Read the model definition and answer for the solid it produces. Units are mm, in the model's axes. Round coordinates to 2 decimals unless told otherwise and drop trailing zeros. Loops run counter-clockwise (first coordinate to the right, second up) from the corner with the lowest first, then second, coordinate; pieces in that order, holes last. Notation, with made-up numbers: M 9,-20.5 L 43,-20.5 A8 cw 43,-9.5 Z; hole C 24.25,-13.5 d1. An arc over 180 degrees is marked long. Write each question's results on one line, items separated by ' | '.
from build123d import *

# Parameters (mm, degrees)
SKETCH2_R           = 2.5
SKETCH2_R_2         = 250
BOSS_EXTRUDE1_DEPTH = 10
CUT_EXTRUDE1_DEPTH  = 11


with BuildPart() as part:
    # Sketch2 → Boss-Extrude1 (new body)
    with BuildSketch(Plane(origin=(0, 0, 0), x_dir=(1, 0, 0), z_dir=(0, 1, 0))):
        with BuildLine():
            Line((-34.517430478, 903.068960265), (-295.040344804, 95.1377682))
            ThreePointArc((-295.040344804, 95.1377682), (-310, 0), (-295.040344804, -95.1377682))
            Line((-295.040344804, -95.1377682), (-34.517430478, -903.068960265))
            ThreePointArc((-34.517430478, -903.068960265), (-30.886866626, -908.083613135), (-25, -910))
            Line((-25, -910), (25, -910))
            ThreePointArc((25, -910), (30.886866626, -908.083613135), (34.517430478, -903.068960265))
            Line((34.517430478, -903.068960265), (295.040344804, -95.1377682))
            ThreePointArc((295.040344804, -95.1377682), (310, 0), (295.040344804, 95.1377682))
            Line((295.040344804, 95.1377682), (34.517430478, 903.068960265))
            ThreePointArc((34.517430478, 903.068960265), (30.886866626, 908.083613135), (25, 910))
            Line((25, 910), (-25, 910))
            ThreePointArc((-25, 910), (-30.886866626, 908.083613135), (-34.517430478, 903.068960265))
        make_face()
        with Locations((-48.373467006, -762.345774842)):
            Circle(SKETCH2_R, mode=Mode.SUBTRACT)
        with Locations((-94.407870974, -619.584317679)):
            Circle(SKETCH2_R, mode=Mode.SUBTRACT)
        with Locations((-140.442274942, -476.822860516)):
            Circle(SKETCH2_R, mode=Mode.SUBTRACT)
        with BuildLine():
            ThreePointArc((-181.680791071, -251.181388952), (0, -310), (181.680791071, -251.181388952))
            Line((181.680791071, -251.181388952), (9.517430478, -785.092770658))
            ThreePointArc((9.517430478, -785.092770658), (0, -792.023810393), (-9.517430478, -785.092770658))
            Line((-9.517430478, -785.092770658), (-181.680791071, -251.181388952))
        make_face(mode=Mode.SUBTRACT)
        with Locations((-186.476678909, -334.061403353)):
            Circle(SKETCH2_R, mode=Mode.SUBTRACT)
        with Locations((48.373467006, -762.345774842)):
            Circle(SKETCH2_R, mode=Mode.SUBTRACT)
        with Locations((94.407870974, -619.584317679)):
            Circle(SKETCH2_R, mode=Mode.SUBTRACT)
        with Locations((140.442274942, -476.822860516)):
            Circle(SKETCH2_R, mode=Mode.SUBTRACT)
        with Locations((186.476678909, -334.061403353)):
            Circle(SKETCH2_R, mode=Mode.SUBTRACT)
        with Locations((-186.476678909, 334.061403353)):
            Circle(SKETCH2_R, mode=Mode.SUBTRACT)
        with Locations((-140.442274942, 476.822860516)):
            Circle(SKETCH2_R, mode=Mode.SUBTRACT)
        with Locations((-94.407870974, 619.584317679)):
            Circle(SKETCH2_R, mode=Mode.SUBTRACT)
        with BuildLine():
            ThreePointArc((181.680791071, 251.181388952), (0, 310), (-181.680791071, 251.181388952))
            Line((-181.680791071, 251.181388952), (-9.517430478, 785.092770658))
            ThreePointArc((-9.517430478, 785.092770658), (0, 792.023810393), (9.517430478, 785.092770658))
            Line((9.517430478, 785.092770658), (181.680791071, 251.181388952))
        make_face(mode=Mode.SUBTRACT)
        with Locations((-48.373467006, 762.345774842)):
            Circle(SKETCH2_R, mode=Mode.SUBTRACT)
        Circle(SKETCH2_R_2, mode=Mode.SUBTRACT)
        with Locations((186.476678909, 334.061403353)):
            Circle(SKETCH2_R, mode=Mode.SUBTRACT)
        with Locations((140.442274942, 476.822860516)):
            Circle(SKETCH2_R, mode=Mode.SUBTRACT)
        with Locations((94.407870974, 619.584317679)):
            Circle(SKETCH2_R, mode=Mode.SUBTRACT)
        with Locations((48.373467006, 762.345774842)):
            Circle(SKETCH2_R, mode=Mode.SUBTRACT)
    extrude(amount=BOSS_EXTRUDE1_DEPTH)

    # Sketch3 → Cut-Extrude1 (cut, through all)
    with BuildSketch(Plane(origin=(0, 10, 0), x_dir=(1, 0, 0), z_dir=(0, 1, 0))):
        Polygon((-49.523523643, -856.532206403), (-40.006093165, -853.463246139), (-70.69569581, -758.288941363), (-80.213126288, -761.357901628), align=None)
        Polygon((-132.074901101, -567.940331812), (-141.592331578, -571.009292077), (-172.281934223, -475.834987302), (-162.764503746, -472.766027037), align=None)
        with BuildLine():
            Line((-233.661139514, -285.486377751), (-224.143709036, -282.417417486))
            Line((-224.143709036, -282.417417486), (-285.522914326, -92.068807935))
            ThreePointArc((-285.522914326, -92.068807935), (-300, 0), (-285.522914326, 92.068807935))
            Line((-285.522914326, 92.068807935), (-224.143709036, 282.417417486))
            Line((-224.143709036, 282.417417486), (-233.661139514, 285.486377751))
            Line((-233.661139514, 285.486377751), (-295.040344804, 95.1377682))
            ThreePointArc((-295.040344804, 95.1377682), (-310, 0), (-295.040344804, -95.1377682))
            Line((-295.040344804, -95.1377682), (-233.661139514, -285.486377751))
        make_face()
        Polygon((-49.523523643, 856.532206403), (-40.006093165, 853.463246139), (-70.69569581, 758.288941363), (-80.213126288, 761.357901628), align=None)
        Polygon((-162.764503746, 472.766027037), (-132.074901101, 567.940331812), (-141.592331578, 571.009292077), (-172.281934223, 475.834987302), align=None)
        Polygon((49.523523643, 856.532206403), (40.006093165, 853.463246139), (70.69569581, 758.288941363), (80.213126288, 761.357901628), align=None)
        Polygon((49.523523643, -856.532206403), (40.006093165, -853.463246139), (70.69569581, -758.288941363), (80.213126288, -761.357901628), align=None)
        Polygon((132.074901101, 567.940331812), (141.592331578, 571.009292077), (172.281934223, 475.834987302), (162.764503746, 472.766027037), align=None)
        with BuildLine():
            Line((233.661139514, 285.486377751), (224.143709036, 282.417417486))
            Line((224.143709036, 282.417417486), (285.522914326, 92.068807935))
            ThreePointArc((285.522914326, 92.068807935), (300, 0), (285.522914326, -92.068807935))
            Line((285.522914326, -92.068807935), (224.143709036, -282.417417486))
            Line((224.143709036, -282.417417486), (233.661139514, -285.486377751))
            Line((233.661139514, -285.486377751), (295.040344804, -95.1377682))
            ThreePointArc((295.040344804, -95.1377682), (310, 0), (295.040344804, 95.1377682))
            Line((295.040344804, 95.1377682), (233.661139514, 285.486377751))
        make_face()
        Polygon((162.764503746, -472.766027037), (132.074901101, -567.940331812), (141.592331578, -571.009292077), (172.281934223, -475.834987302), align=None)
    extrude(amount=-CUT_EXTRUDE1_DEPTH, mode=Mode.SUBTRACT)


solid = part.part
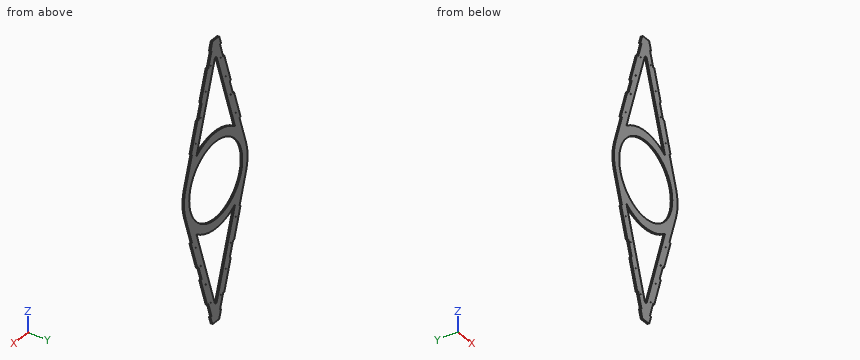
Item 1: The part is cut by section B-B (z = -660). Determine the outline of the cut face in (x, y).
Outcome:
outline: M -112.9,0 L -49.85,0 L -49.85,10 L -112.9,10 Z; M 49.85,0 L 112.9,0 L 112.9,10 L 49.85,10 Z
Item 2: The part is cut by section A-A (z = 0). Determine the outline of the cut face in (x, y), plus the area to 3 significant figures.
Outcome:
outline: M -300,0 L -250,0 L -250,10 L -300,10 Z; M 250,0 L 300,0 L 300,10 L 250,10 Z | area: 1,000 mm2
Item 3: The part is cut by section C-C (y = 2.75). State how many separate pieces and enclosed holes the cut face has, plus the area to 3 significant figures.
Outcome:
separate pieces: 1 | enclosed holes: 19 | area: 258,000 mm2
Item 4: Straight lines are drawn through the part: line 1 (X direction, y = 1, z = -4.5); line 2 (X direction, y = 2.75, z = -255.5); line 3 (X direction, y = 8, z = -333). For each, find the intervals that lie inside material, in ascending order.
Outcome:
line 1: x = -299.97 to -249.96, 249.96 to 299.97 | line 2: x = -232.82 to -180.29, -175.56 to 175.56, 180.29 to 232.82 | line 3: x = -218.34 to -188.74, -184.21 to -155.3, 155.3 to 184.21, 188.74 to 218.34
Item 5: Flat-ended cylindrical pins translate along their axes: pin 1 (6.5 mm diameter, centred on x = 186.48, z = -334.06, fed in from +Y); pin 2 (3 mm diameter, centred on x = -140.44, z = 476.82, fed in from -Y); pin 3 (3 mm diameter, centred on y = 5, z = 72, fed in from -X). Find the tip coordinate at first contact, or state that the pin passes through.
Outcome:
pin 1: stops at y = 10 | pin 2: passes through | pin 3: stops at x = -291.6
